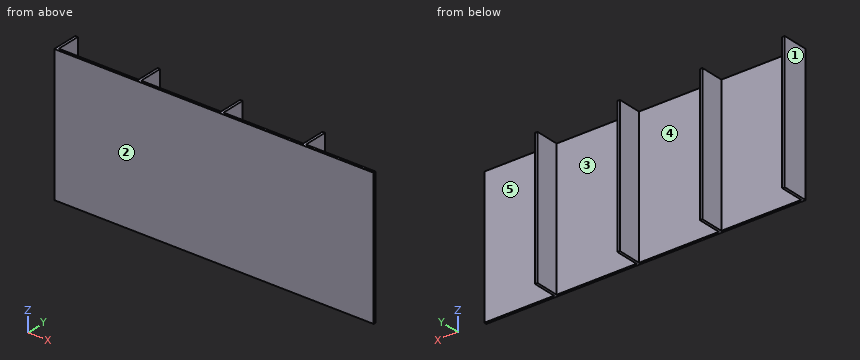
Autodesk Inventor part; units mm, degrees
ref_plane "YZ Plane" through (0, 0, 0) normal (1, 0, 0) x (0, 1, 0)
ref_plane "XZ Plane" through (0, 0, 0) normal (0, 1, 0) x (-1, 0, 0)
ref_plane "XY Plane" through (0, 0, 0) normal (0, 0, 1) x (1, 0, 0)
sketch "Sketch1" plane through (0, 0, 0) normal (0, 0, 1) x (1, 0, 0)
  line L0 (0, 0) -> (-203.2, 0)
  line L1 (-203.2, 0) -> (-203.2, -1.6002)
  line L2 (-203.2, -1.6002) -> (0, -1.6002)
  line L3 (0, -1.6002) -> (0, 0)
  dimension "d0" = 203.2
  dimension "d1" = 1.6002
extrude "Extrusion1" add sketch "Sketch1" along normal blind 86.36
sketch "Sketch2" plane through (-203.2, 0, 0) normal (0, 1, 0) x (1, 0, 0)
  line L0 (203.2, 0) -> (0, 0)
  line L1 (203.2, -86.36) -> (0, -86.36)
  line L2 (0, 0) -> (1.6002, 0)
  line L3 (1.6002, 0) -> (1.6002, -86.36)
  line L4 (1.6002, -86.36) -> (0, -86.36)
  line L5 (0, -86.36) -> (0, 0)
  dimension "d4" = 1.6002
extrude "Extrusion2" add sketch "Sketch2" along normal blind 15.24
sketch "Sketch3" plane through (0, 0, 86.36) normal (0, 1, 0) x (1, 0, 0)
  line L0 (-203.2, 0) -> (0, 0)
  line L1 (-203.2, 86.36) -> (0, 86.36)
  line L2 (-150.7998, 0) -> (-149.1996, 0)
  line L3 (-149.1996, 0) -> (-149.1996, 86.36)
  line L4 (-149.1996, 86.36) -> (-150.7998, 86.36)
  line L5 (-150.7998, 86.36) -> (-150.7998, 0)
  dimension "d7" = 1.6002
extrude "Extrusion3" add sketch "Sketch3" along normal blind 15.24
sketch "Sketch4" plane through (0, 0, 86.36) normal (0, 1, 0) x (1, 0, 0)
  line L0 (-203.2, 0) -> (0, 0)
  line L1 (-203.2, 86.36) -> (0, 86.36)
  line L2 (-98.3996, 0) -> (-96.7994, 0)
  line L3 (-96.7994, 0) -> (-96.7994, 86.36)
  line L4 (-96.7994, 86.36) -> (-98.3996, 86.36)
  line L5 (-98.3996, 86.36) -> (-98.3996, 0)
  dimension "d10" = 1.6002
extrude "Extrusion4" add sketch "Sketch4" along normal blind 15.24
sketch "Sketch5" plane through (0, 0, 86.36) normal (0, 1, 0) x (1, 0, 0)
  line L0 (0, 0) -> (-96.7994, 0)
  line L1 (0, 86.36) -> (-96.7994, 86.36)
  line L2 (-45.9994, 0) -> (-44.3992, 0)
  line L3 (-44.3992, 0) -> (-44.3992, 86.36)
  line L4 (-44.3992, 86.36) -> (-45.9994, 86.36)
  line L5 (-45.9994, 86.36) -> (-45.9994, 0)
  dimension "d13" = 1.6002
extrude "Extrusion5" add sketch "Sketch5" along normal blind 15.24
properties part number "ModulePlate2.0"
Could you check a few things on this model? Use its own coordinates, in mm. Face numbers are marked on the shaded views. A direction names the side the tool comes from. Round coordinates to 2 decimals unless told otherwise and drop trailing zeros. Loops run counter-clockwise (first coordinate to the right, second up) from the corner with the lowest first, then second, coordinate; pieces in that order, holes last.
Q1. For P1, Ø7.5, axis at y = 9, z = 28, coming from the +X side; P2, Ø8, axis at x = -135, y = 7, coming from the +Z side; P3, Ø8, axis at x = -82.5, z = 16, coming from the +Y side, each with a flat end and sliding along its axis, tell me the tip position at first contact or that it passes through.
Q2. I want a section at B-B (z = 50). Write out the boundary of the cut face in (x, y).
Q3. I want a section at C-C (x = -41). Write out the boundary of the cut face in (y, z).
Q4. Thinking about a two-plate mould opening in X: for the marked faces 1, 2 and 3, which applies, pulls with the +X half, pulls with the -X half, needs draft (parallel to the pull), parting line crosses it, or undercut?
Q5. On a 3-axis mill with a long thin cutter (end or side, diameter ignored), from which of +Z, -Z, +X, -X, +Y, -Y can I reach the whole of each face in a straight line? I mean the marked faces 4 and 5. Say none if no direction works.
Q6. I want a section at A-A (y = 5.75). Write out the boundary of the cut face in (x, z).
Q7. Please list where these lines run through material, in increasing order: L1, parallel to X at y = 12.25, z = 38; L2, parallel to Y at x = -130, z = 32.5.
Answer below:
1. P1: stops at x = -44.4
1. P2: passes through
1. P3: stops at y = 0
2. outline: (-203.2, -1.6) - (0, -1.6) - (0, 0) - (-44.4, 0) - (-44.4, 15.24) - (-46, 15.24) - (-46, 0) - (-96.8, 0) - (-96.8, 15.24) - (-98.4, 15.24) - (-98.4, 0) - (-149.2, 0) - (-149.2, 15.24) - (-150.8, 15.24) - (-150.8, 0) - (-201.6, 0) - (-201.6, 15.24) - (-203.2, 15.24) - close
3. outline: (-1.6, 0) - (0, 0) - (0, 86.36) - (-1.6, 86.36) - close
4. face 1: pulls with the -X half
4. face 2: needs draft
4. face 3: undercut
5. face 4: +Z, -Z, +Y
5. face 5: +Z, -Z, +X, +Y
6. outline: (-203.2, 0) - (-201.6, 0) - (-201.6, 86.36) - (-203.2, 86.36) - close; (-150.8, 0) - (-149.2, 0) - (-149.2, 86.36) - (-150.8, 86.36) - close; (-98.4, 0) - (-96.8, 0) - (-96.8, 86.36) - (-98.4, 86.36) - close; (-46, 0) - (-44.4, 0) - (-44.4, 86.36) - (-46, 86.36) - close
7. L1: x = -203.2 to -201.6, -150.8 to -149.2, -98.4 to -96.8, -46 to -44.4
7. L2: y = -1.6 to 0
